Geometry check sheet. Reference: the model listing, model coordinates, mm. Face numbers are marked on the shaded views. A direction names the side the tool comes from. Give positions to 0.01 mm unless a question says otherwise; leave off trailing zeros. Order: outer loops, then holes, each group sorted by start corner. A loop starts at its lowest first (then second) coordinate and runs counter-clockwise, first axis right, second up.
from build123d import *

# Parameters (mm, degrees)
COILBASE_R                     = 7.25
BOSS_EXTRUDE1_DEPTH            = 28.575
WIREHOUSING_EXTRUDE_DEPTH      = 5
WIREHOUSING_EXTRUDE_DEPTH_BACK = 5
WIREHOUSING_R                  = 8.25
BOSS_EXTRUDE3_DEPTH            = 17.2875
BOSS_EXTRUDE3_DEPTH_BACK       = 17.2875
CLEARANCEFORACTUATOR_R         = 3


with BuildPart() as part:
    # CoilBase → Boss-Extrude1 (new body)
    with BuildSketch(Plane(origin=(0, 0, 0), x_dir=(0, 0, -1), z_dir=(1, 0, 0))):
        Circle(COILBASE_R)
    extrude(amount=BOSS_EXTRUDE1_DEPTH)

    # WireHousing → WireHousing-Extrude (add, two sides: drawn at the far end of the back side and taken through both)
    with BuildSketch(Plane(origin=(14.29, 0, 0), x_dir=(0, 0, -1), z_dir=(1, 0, 0)).offset(-WIREHOUSING_EXTRUDE_DEPTH_BACK)):
        Circle(WIREHOUSING_R)
    extrude(amount=WIREHOUSING_EXTRUDE_DEPTH + WIREHOUSING_EXTRUDE_DEPTH_BACK)

    # ClearanceForActuator → Boss-Extrude3 (add, two sides: drawn at the far end of the back side and taken through both)
    with BuildSketch(Plane(origin=(14.29, 0, 0), x_dir=(0, 0, -1), z_dir=(1, 0, 0)).offset(-BOSS_EXTRUDE3_DEPTH_BACK)):
        Circle(CLEARANCEFORACTUATOR_R)
    extrude(amount=BOSS_EXTRUDE3_DEPTH + BOSS_EXTRUDE3_DEPTH_BACK)


solid = part.part
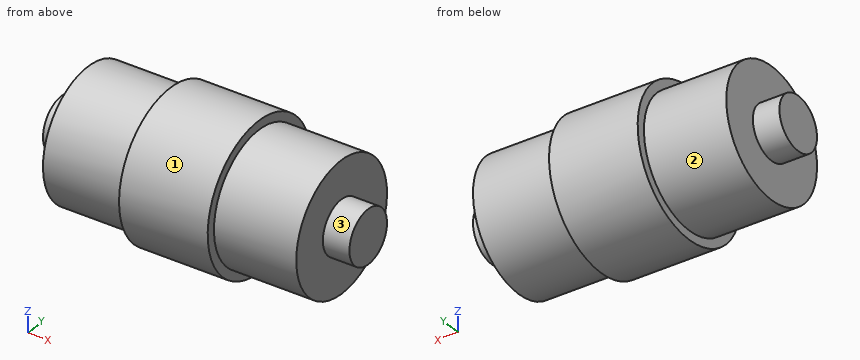
Item 1: Sectioned sample at D-D (y = 5.5). Enter the section's corners in (x, z) (3 decimals), and give its area (3 significant figures).
Reported:
outline: (0, -4.724) - (9.29, -4.724) - (9.29, -6.149) - (19.29, -6.149) - (19.29, -4.724) - (28.575, -4.724) - (28.575, 4.724) - (19.29, 4.724) - (19.29, 6.149) - (9.29, 6.149) - (9.29, 4.724) - (0, 4.724) - close
area: 298 mm2
Item 2: Sectioned sample at C-C (x = 16.5). Enter the section's corners in (y, z).
Reported:
outline: circle Ø16.5 at (0, 0)
Item 3: Sectioned sample at B-B (y = 1.25). Enter the section's corners in (x, z) (1 decimal).
Reported:
outline: (-3, -2.7) - (0, -2.7) - (0, -7.1) - (9.3, -7.1) - (9.3, -8.2) - (19.3, -8.2) - (19.3, -7.1) - (28.6, -7.1) - (28.6, -2.7) - (31.6, -2.7) - (31.6, 2.7) - (28.6, 2.7) - (28.6, 7.1) - (19.3, 7.1) - (19.3, 8.2) - (9.3, 8.2) - (9.3, 7.1) - (0, 7.1) - (0, 2.7) - (-3, 2.7) - close
Item 4: Scan lines: L1, parallel to X at y = -2, z = 5.25 (3 decimals); L2, parallel to Z at x = 6, y = -0.25; L3, parallel to Z at x = 17, y = -4.5. Record each from-to range of solid material in increasing order.
Reported:
L1: x = 0 to 28.575
L2: z = -7.25 to 7.25
L3: z = -6.91 to 6.91
Item 5: Gauge pin test, flat ends, axial feed: pin 1 (1.5 mm diameter, centred on y = 5.5, z = -0.5, fed in from +X) (3 decimals); pin 2 (6 mm diameter, centred on x = 1.5, z = -0.5, fed in from +Y). Record the tip position at first contact, or that the pin passes through.
Reported:
pin 1: stops at x = 28.575
pin 2: stops at y = 7.25
Item 6: Set-up check for the marked faces 1, 2 and 3: record each of +Z, -Z, +X, -X, +Y, -Y from which the full face is reachable in a straight line by a thin tool's end or side.
Reported:
face 1: +X, -X
face 2: -X
face 3: +X
